Geometry: final body of the model. Coordinates: model frame, mm. A direction names the side the tool comes from. Give positions to 0.01 mm unless a question says otherwise; leave off trailing zeros. Write each loop counter-clockwise with the first axis right and the second up, starting at its lowest first coordinate (ties: lowest second). Pieces come first, ordered by that corner, then holes.
Q1. Line query: line 1 (Z direction, x = -101, y = 9.75); line 2 (X direction, y = 18.8, z = 0); line 3 (X direction, y = 12.5, z = 0). Output: solid intervals per line, ascending.
Q2. Section C-C (x = -83.5). Return the cut outline in (y, z).
Q3. Section A-A (x = 0). Return the cut outline in (y, z), plus the area to 3 significant figures.
Q4. Section B-B (z = 0). Return the cut outline in (x, y).
Q5. Mould query, pull axis Z, two halves, no side actions, for faces 1 (the flat face through (-2, 11, 100.33)), 2 (the flat face through (-122, 14, 65.151)), 3 (the flat face through (-125.412, 11, -1)). Classes: +Z half, -Z half, draft (parallel to the pull), parting line (faces both ways), or undercut.
Q6. Reachability of faces 4 (the flat face through (125.412, 11, 1)), 5 (the flat face through (-2, 0, -68)), 6 (the flat face through (-111, 6.223, 44)), 7 (the flat face through (118.821, 14, 60)), 8 (the flat face through (-99.86, 17, -98)) from +Z, -Z, +X, -X, +Y, -Y: full face, straight path, thin tool, end or side. Return the list, or none.
Q7. Pin query (flat end, axial travel): pin 1 Ø4.5 at (x, z) = (-120.5, -74) entering from +Y; pin 2 Ø6 at (x, z) = (-32, -69) entering from +Y; pin 3 Ø11.5 at (y, z) = (14.5, 29.5) entering from +X. Return the tip coordinate at first contact, or that it passes through.
from build123d import *

# Parameters (mm, degrees)
BOSS_EXTRUDE1_DEPTH     = 21.463
SKETCH3_R               = 88.9
CUT_EXTRUDE1_DEPTH      = 5.0546
CUT_EXTRUDE2_DEPTH      = 162.442372526
CUT_EXTRUDE2_DEPTH_BACK = 162.442372526
SKETCH4_R               = 64.5033
SKETCH5_W               = 250.825
SKETCH5_H               = 200.66
BOSS_EXTRUDE2_DEPTH     = 6.223
CUT_EXTRUDE3_DEPTH      = 162.442372526
CUT_EXTRUDE3_DEPTH_BACK = 162.442372526
SKETCH4_2_R             = 64.5033
SKETCH6_W               = 6.604
SKETCH6_H               = 5.0038
SKETCH6_W_2             = 7.62
SKETCH6_H_2             = 6.604
CUT_EXTRUDE4_DEPTH      = 11.176
FILLET4_R               = 1.27


with BuildPart() as part:
    # Sketch2 → Boss-Extrude1 (new body)
    with BuildSketch(Plane(origin=(0, 0, 0), x_dir=(1, 0, 0), z_dir=(0, 1, 0))):
        with BuildLine():
            Line((-125.4125, 65.151), (-119.0752, 65.151))
            ThreePointArc((-119.0752, 65.151), (-118.895594878, 65.076605122), (-118.8212, 64.897))
            Line((-118.8212, 64.897), (-118.8212, 54.4195))
            ThreePointArc((-118.8212, 54.4195), (-118.746805122, 54.239894878), (-118.5672, 54.1655))
            Line((-118.5672, 54.1655), (-87.8713, 54.1655))
            ThreePointArc((-87.8713, 54.1655), (-87.691694878, 54.091105122), (-87.6173, 53.9115))
            Line((-87.6173, 53.9115), (-87.6173, 34.0995))
            ThreePointArc((-87.6173, 34.0995), (-87.691694878, 33.919894878), (-87.8713, 33.8455))
            Line((-87.8713, 33.8455), (-118.5672, 33.8455))
            ThreePointArc((-118.5672, 33.8455), (-118.746805122, 33.771105122), (-118.8212, 33.5915))
            Line((-118.8212, 33.5915), (-118.8212, 23.114))
            ThreePointArc((-118.8212, 23.114), (-118.895594878, 22.934394878), (-119.0752, 22.86))
            Line((-119.0752, 22.86), (-125.4125, 22.86))
            Line((-125.4125, 22.86), (-125.4125, -22.86))
            Line((-125.4125, -22.86), (-119.0752, -22.86))
            ThreePointArc((-119.0752, -22.86), (-118.895594878, -22.934394878), (-118.8212, -23.114))
            Line((-118.8212, -23.114), (-118.8212, -33.5915))
            ThreePointArc((-118.8212, -33.5915), (-118.746805122, -33.771105122), (-118.5672, -33.8455))
            Line((-118.5672, -33.8455), (-87.8713, -33.8455))
            ThreePointArc((-87.8713, -33.8455), (-87.691694878, -33.919894878), (-87.6173, -34.0995))
            Line((-87.6173, -34.0995), (-87.6173, -53.9115))
            ThreePointArc((-87.6173, -53.9115), (-87.691694878, -54.091105122), (-87.8713, -54.1655))
            Line((-87.8713, -54.1655), (-118.5672, -54.1655))
            ThreePointArc((-118.5672, -54.1655), (-118.746805122, -54.239894878), (-118.8212, -54.4195))
            Line((-118.8212, -54.4195), (-118.8212, -64.897))
            ThreePointArc((-118.8212, -64.897), (-118.895594878, -65.076605122), (-119.0752, -65.151))
            Line((-119.0752, -65.151), (-125.4125, -65.151))
            Line((-125.4125, -65.151), (-125.4125, -100.33))
            Line((-125.4125, -100.33), (125.4125, -100.33))
            Line((125.4125, -100.33), (125.4125, -65.151))
            Line((125.4125, -65.151), (119.0752, -65.151))
            ThreePointArc((119.0752, -65.151), (118.895594878, -65.076605122), (118.8212, -64.897))
            Line((118.8212, -64.897), (118.8212, -54.4195))
            ThreePointArc((118.8212, -54.4195), (118.746805122, -54.239894878), (118.5672, -54.1655))
            Line((118.5672, -54.1655), (87.8713, -54.1655))
            ThreePointArc((87.8713, -54.1655), (87.691694878, -54.091105122), (87.6173, -53.9115))
            Line((87.6173, -53.9115), (87.6173, -34.0995))
            ThreePointArc((87.6173, -34.0995), (87.691694878, -33.919894878), (87.8713, -33.8455))
            Line((87.8713, -33.8455), (118.5672, -33.8455))
            ThreePointArc((118.5672, -33.8455), (118.746805122, -33.771105122), (118.8212, -33.5915))
            Line((118.8212, -33.5915), (118.8212, -23.114))
            ThreePointArc((118.8212, -23.114), (118.895594878, -22.934394878), (119.0752, -22.86))
            Line((119.0752, -22.86), (125.4125, -22.86))
            Line((125.4125, -22.86), (125.4125, 22.86))
            Line((125.4125, 22.86), (119.0752, 22.86))
            ThreePointArc((119.0752, 22.86), (118.895594878, 22.934394878), (118.8212, 23.114))
            Line((118.8212, 23.114), (118.8212, 33.5915))
            ThreePointArc((118.8212, 33.5915), (118.746805122, 33.771105122), (118.5672, 33.8455))
            Line((118.5672, 33.8455), (87.8713, 33.8455))
            ThreePointArc((87.8713, 33.8455), (87.691694878, 33.919894878), (87.6173, 34.0995))
            Line((87.6173, 34.0995), (87.6173, 53.9115))
            ThreePointArc((87.6173, 53.9115), (87.691694878, 54.091105122), (87.8713, 54.1655))
            Line((87.8713, 54.1655), (118.5672, 54.1655))
            ThreePointArc((118.5672, 54.1655), (118.746805122, 54.239894878), (118.8212, 54.4195))
            Line((118.8212, 54.4195), (118.8212, 64.897))
            ThreePointArc((118.8212, 64.897), (118.895594878, 65.076605122), (119.0752, 65.151))
            Line((119.0752, 65.151), (125.4125, 65.151))
            Line((125.4125, 65.151), (125.4125, 100.33))
            Line((125.4125, 100.33), (-125.4125, 100.33))
            Line((-125.4125, 100.33), (-125.4125, 65.151))
        make_face()
    extrude(amount=BOSS_EXTRUDE1_DEPTH)

    # Sketch3 → Cut-Extrude1 (cut)
    with BuildSketch(Plane(origin=(0, 21.463, 0), x_dir=(1, 0, 0), z_dir=(0, 1, 0))):
        with Locations(Location((0, 0, 0), (0, 0, 270))):
            Circle(SKETCH3_R)
    extrude(amount=-CUT_EXTRUDE1_DEPTH, mode=Mode.SUBTRACT)

    # Sketch4 → Cut-Extrude2 (cut, two sides: drawn at the far end of the back side and taken through both)
    with BuildSketch(Plane(origin=(0, 16.4084, 0), x_dir=(1, 0, 0), z_dir=(0, 1, 0)).offset(-CUT_EXTRUDE2_DEPTH_BACK)):
        with Locations(Location((0, 0, 0), (0, 0, 270))):
            Circle(SKETCH4_R)
    extrude(amount=CUT_EXTRUDE2_DEPTH + CUT_EXTRUDE2_DEPTH_BACK, mode=Mode.SUBTRACT)

    # Sketch5 → Boss-Extrude2 (add)
    with BuildSketch(Plane.XZ):
        Rectangle(SKETCH5_W, SKETCH5_H)
    extrude(amount=-BOSS_EXTRUDE2_DEPTH)

    # Sketch4_2 → Cut-Extrude3 (cut, two sides: drawn at the far end of the back side and taken through both)
    with BuildSketch(Plane(origin=(0, 16.4084, 0), x_dir=(1, 0, 0), z_dir=(0, 1, 0)).offset(-CUT_EXTRUDE3_DEPTH_BACK)):
        with Locations(Location((0, 0, 0), (0, 0, 270))):
            Circle(SKETCH4_2_R)
    extrude(amount=CUT_EXTRUDE3_DEPTH + CUT_EXTRUDE3_DEPTH_BACK, mode=Mode.SUBTRACT)

    # Sketch6 → Cut-Extrude4 (cut)
    with BuildSketch(Plane(origin=(0, 21.463, 0), x_dir=(1, 0, 0), z_dir=(0, 1, 0))):
        with Locations((-103.1621, 97.8281)):
            Rectangle(SKETCH6_W, SKETCH6_H)
        with Locations((-121.6025, 74.7776)):
            Rectangle(SKETCH6_W_2, SKETCH6_H_2)
    extrude(amount=-CUT_EXTRUDE4_DEPTH, mode=Mode.SUBTRACT)

    # Fillet4
    fillet4_edges = [part.edges().sort_by_distance(p)[0] for p in [
        (-106.4641, 10.287, -97.8281),
        (-99.8601, 10.287, -97.8281),
        (-121.6025, 10.287, -78.0796),
        (-121.6025, 10.287, -71.4756),
    ]]
    fillet(fillet4_edges, radius=FILLET4_R)


solid = part.part
Computed:
1. line 1: z = -100.33 to -54.17, -33.85 to 33.85, 54.17 to 100.33
1. line 2: x = -125.41 to -88.9, 88.9 to 125.41
1. line 3: x = -125.41 to -64.5, 64.5 to 125.41
2. outline: (0, -100.33) - (21.46, -100.33) - (21.46, -30.51) - (16.41, -30.51) - (16.41, 30.51) - (21.46, 30.51) - (21.46, 100.33) - (0, 100.33) - close
3. outline: (0, -100.33) - (21.46, -100.33) - (21.46, -88.9) - (16.41, -88.9) - (16.41, -64.5) - (0, -64.5) - close; (0, 64.5) - (16.41, 64.5) - (16.41, 88.9) - (21.46, 88.9) - (21.46, 100.33) - (0, 100.33) - close
3. area: 1,290 mm2
4. outline: (-125.41, 0) - (-64.5, 0) - (-64.5, 16.41) - (-88.9, 16.41) - (-88.9, 21.46) - (-125.41, 21.46) - close; (64.5, 0) - (125.41, 0) - (125.41, 21.46) - (88.9, 21.46) - (88.9, 16.41) - (64.5, 16.41) - close
5. face 1: +Z half
5. face 2: undercut
5. face 3: draft
6. face 4: +Z, -Z, +X, +Y, -Y
6. face 5: +Z, -Z, +X, -X, -Y
6. face 6: -X, +Y
6. face 7: +X, +Y
6. face 8: -Z, +Y
7. pin 1: stops at y = 10.77
7. pin 2: stops at y = 16.41
7. pin 3: stops at x = 118.82
